Verification items for the finished model (mm, model axes). A direction names the side the tool comes from. Coordinates: 2 decimals unless noted, no trailing zeros. Loops run counter-clockwise (first coordinate to the right, second up) from the corner with the lowest first, then second, coordinate; pieces in that order, holes last. Notation, with made-up numbers: (18.25, -14.75) -> (62.25, -14.75) arc R21 ccw to (62.25, 6.25) -> close; hole circle Ø1 at (43, 71). An arc over 180 degrees is marked (long way). Answer as a JSON object with one key per item and string values. Group by question number.
Q1. Cross-section at C-C on y = 0. Give the number of separate pieces and of enclosed holes in the cut face, and give its area (3 significant figures).
Q2. Release check for a two-part mould opening along X. For faces 4 (the cylindrical face through (-22.5, 0.1, 1.4)), 5 (the flat face through (-13, -1, 0)), 6 (the cylindrical face through (10.5, 0.05, 1.23)), 7 (the flat face through (-0.27, -3.15, 3.39)) record: released by +X, released by -X, zero draft, split by the parting line, or undercut.
Q3. Set-up check for faces 1 (the flat face through (-13, 1, 2.5)), 2 (the cylindrical face through (15.25, 0.08, -0.99)), 3 (the flat face through (10.6, -0.8, 0)): record each of +Z, -Z, +X, -X, +Y, -Y from which the full face is reachable in a straight line by a thin tool's end or side.
Q4. Cross-section at D-D on x = -8.5. Record the boundary of the cut face in (y, z).
Q5. Cross-section at A-A on z = 2.1. Record the boundary of the cut face in (x, y), and give its area (3 significant figures).
Q6. Gauge pin test, flat ends, axial feed: pin 1 Ø3 at (x, y) = (11.75, 0) entering from +Z; pin 2 Ø2 at (y, z) = (2, 2) entering from +X; pin 3 Ø4 at (x, y) = (11.75, 0) entering from -Z; pin 4 Ø3 at (x, y) = (-11.75, 0) entering from -Z. Record the tip position at first contact, or that the pin passes through.
Q7. Scan lines: L1, parallel to Y at x = 11.75, z = 0.5; L2, parallel to X at y = 0.5, z = -1.35; L3, parallel to X at y = 1.25, z = -0.6. Record each from-to range of solid material in increasing order.
Q8. Cross-section at B-B on x = -16. Record the boundary of the cut face in (y, z).
```python
from build123d import *

# Parameters (mm, degrees)
SKETCH1_W           = 38
SKETCH1_H           = 7
SKETCH1_R           = 1.25
BOSS_EXTRUDE1_DEPTH = 4
CHAMFER1_SIZE       = 0.7
CHAMFER1_SIZE2      = 1.212435565
SKETCH2_R           = 1.78594
BOSS_EXTRUDE2_DEPTH = 2
SKETCH3_R           = 1.25
CUT_EXTRUDE1_DEPTH  = 3.5
SKETCH4_R           = 1.78594
CUT_EXTRUDE2_DEPTH  = 1.5


with BuildPart() as part:
    # Sketch1 → Boss-Extrude1 (new body)
    # profile 1 of 3: a face of its own
    with BuildSketch(Plane.XY):
        Rectangle(SKETCH1_W, SKETCH1_H)
        with Locations((11.75, 0)):
            Circle(SKETCH1_R, mode=Mode.SUBTRACT)
        with Locations((-11.75, 0)):
            Circle(SKETCH1_R, mode=Mode.SUBTRACT)
    # profile 2 of 3: a face of its own
    with BuildSketch(Plane.XY):
        with BuildLine():
            Line((-19, -3.5), (-19, 3.5))
            ThreePointArc((-19, 3.5), (-22.5, 0), (-19, -3.5))
        make_face()
    # profile 3 of 3: a face of its own
    with BuildSketch(Plane.XY):
        with BuildLine():
            ThreePointArc((19, 3.5), (22.5, 0), (19, -3.5))
            Line((19, -3.5), (19, 3.5))
        make_face()
    extrude(amount=BOSS_EXTRUDE1_DEPTH)

    # Chamfer1
    chamfer1_edges = [part.edges().sort_by_distance(p)[0] for p in [
        (0, -3.5, 4),
        (22.5, 0, 4),
        (0, 3.5, 4),
        (-22.5, 0, 4),
    ]]
    chamfer1_side = [part.faces().sort_by_distance(p)[0] for p in [
        (0, 0, 4),
    ]]
    chamfer(chamfer1_edges, length=CHAMFER1_SIZE, length2=CHAMFER1_SIZE2, reference=chamfer1_side[0])

    # Sketch2 → Boss-Extrude2 (add)
    with BuildSketch(Plane(origin=(0, 0, 0), x_dir=(-1, 0, 0), z_dir=(0, 0, -1))):
        with BuildLine():
            ThreePointArc((-11.75, 3.5), (-15.25, 0), (-11.75, -3.5))
            Line((-11.75, -3.5), (11.75, -3.5))
            ThreePointArc((11.75, -3.5), (15.25, 0), (11.75, 3.5))
            Line((11.75, 3.5), (-11.75, 3.5))
        make_face()
        with Locations((-11.75, 0)):
            Circle(SKETCH2_R, mode=Mode.SUBTRACT)
        with Locations((11.75, 0)):
            Circle(SKETCH2_R, mode=Mode.SUBTRACT)
    extrude(amount=BOSS_EXTRUDE2_DEPTH)

    # Sketch3 → Cut-Extrude1 (cut)
    with BuildSketch(Plane(origin=(0, 0, 0), x_dir=(-1, 0, 0), z_dir=(0, 0, -1))):
        with Locations((-19, 0)):
            Circle(SKETCH3_R)
        with Locations((19, 0)):
            Circle(SKETCH3_R)
    extrude(amount=-CUT_EXTRUDE1_DEPTH, mode=Mode.SUBTRACT)

    # Sketch4 → Cut-Extrude2 (cut)
    with BuildSketch(Plane.XY.offset(4)):
        with Locations(Location((-11.75, 0, 0), (0, 0, 180))):
            Circle(SKETCH4_R)
        with Locations(Location((11.75, 0, 0), (0, 0, 180))):
            Circle(SKETCH4_R)
    extrude(amount=-CUT_EXTRUDE2_DEPTH, mode=Mode.SUBTRACT)


solid = part.part
```
Computed values:
{
 "1": {"separate pieces": "3", "enclosed holes": "0", "area": "185 mm²"},
 "2": {"face 4": "released by -X", "face 5": "undercut", "face 6": "undercut", "face 7": "zero draft"},
 "3": {"face 1": "+Z", "face 2": "-Z, +X", "face 3": "-Z"},
 "4": {"outline": "(-3.5, -2) -> (3.5, -2) -> (3.5, 2.79) -> (2.8, 4) -> (-2.8, 4) -> (-3.5, 2.79) -> close"},
 "5": {"outline": "(-19, -3.5) -> (19, -3.5) arc R3.5 ccw to (19, 3.5) -> (-19, 3.5) arc R3.5 ccw to start; hole circle Ø2.5 at (-19, 0); hole circle Ø2.5 at (-11.75, 0); hole circle Ø2.5 at (11.75, 0); hole circle Ø2.5 at (19, 0)", "area": "285 mm²"},
 "6": {"pin 1": "stops at z = 2.5", "pin 2": "stops at x = 22.35", "pin 3": "stops at z = -2", "pin 4": "stops at z = 0"},
 "7": {"L1": "y = -3.5 to -1.25, 1.25 to 3.5", "L2": "x = -15.21 to -13.46, -10.04 to 10.04, 13.46 to 15.21", "L3": "x = -15.02 to -13.03, -10.47 to 10.47, 13.03 to 15.02"},
 "8": {"outline": "(-3.5, 0) -> (3.5, 0) -> (3.5, 2.79) -> (2.8, 4) -> (-2.8, 4) -> (-3.5, 2.79) -> close"}
}
